Input: part model. Units: mm. Frame: model coordinates. Face numbers are marked on the shaded views. A direction names the side the tool comes from. Round coordinates to 2 decimals unless told otherwise and drop trailing zeros. Write each loop counter-clockwise with the first axis right and the second up, starting at its lowest first coordinate (ties: lowest second). Pieces come first, ordered by that corner, then holes. Notation, with made-up numbers: (75.25, 61) - (102.25, 61) arc R13 cw to (102.25, 69) - close; hole circle Ø5 at (22, 51.25). An arc over 180 degrees is marked (long way). Use one line per item in the form item = value.
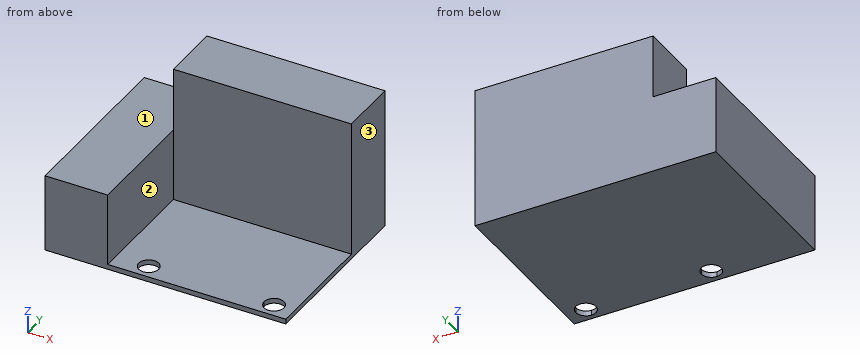
```python
from build123d import *

# Parameters (mm, degrees)
F1_DEPTH = 14.5
F0_W     = 35.5
F0_H     = 12
F2_DEPTH = 27.2
F3_DEPTH = 1


with BuildPart() as f1:
    # F0 (on Top) → F1 (new body)
    with BuildSketch(Plane.XY):
        Polygon((-24, -17.75), (-11.5, -17.75), (-11.5, -16.75), (-11.5, 5.75), (-11.5, 17.75), (-24, 17.75), align=None)
    extrude(amount=F1_DEPTH)

    # F0 (on Top) → F2 (join)
    with BuildSketch(Plane.XY):
        with Locations((6.25, 11.75)):
            Rectangle(F0_W, F0_H)
    extrude(amount=F2_DEPTH)

    # F0 (on Top) → F3 (join)
    with BuildSketch(Plane.XY):
        with Locations((6.25, 11.75)):
            Rectangle(F0_W, F0_H)
        Polygon((-11.5, -17.75), (24, -17.75), (24, -16.75), (20, -16.75), (-5, -16.75), (-11.5, -16.75), align=None)
        Polygon((-24, -17.75), (-11.5, -17.75), (-11.5, -16.75), (-11.5, 5.75), (-11.5, 17.75), (-24, 17.75), align=None)
        with BuildLine():
            Line((-11.5, 5.75), (-11.5, -16.75))
            Line((-11.5, -16.75), (-5, -16.75))
            ThreePointArc((-5, -16.75), (-6.4142135624, -13.3357864376), (-3, -14.75))
            Line((-3, -14.75), (18, -14.75))
            ThreePointArc((18, -14.75), (20, -12.75), (22, -14.75))
            Line((22, -14.75), (24, -14.75))
            Line((24, -14.75), (24, 5.75))
            Line((24, 5.75), (-11.5, 5.75))
        make_face()
        with BuildLine():
            Line((-5, -16.75), (20, -16.75))
            ThreePointArc((20, -16.75), (18.5857864376, -16.1642135624), (18, -14.75))
            Line((18, -14.75), (-3, -14.75))
            ThreePointArc((-3, -14.75), (-3.5857864376, -16.1642135624), (-5, -16.75))
        make_face()
        with BuildLine():
            Line((20, -16.75), (24, -16.75))
            Line((24, -16.75), (24, -14.75))
            Line((24, -14.75), (22, -14.75))
            ThreePointArc((22, -14.75), (21.4142135624, -16.1642135624), (20, -16.75))
        make_face()
    extrude(amount=-F3_DEPTH)


solid = f1.part
```
(1) First-contact query: pin 1 Ø3 at (x, z) = (-7, 22.5) entering from -Y; pin 2 Ø13 at (y, z) = (14.5, 23) entering from -X; pin 3 Ø7 at (y, z) = (-7.5, 9) entering from +X. Flat tips, straight axial feed; report the tip coordinate or a pass-through.
Derived:
pin_1 = 5.75
pin_2 = -11.5
pin_3 = -11.5
(2) Cut plane A-A on y = -10. Output: boundary loops of the cut face in (x, z), then the cut area to 3 significant figures.
Derived:
outline = (-24, -1) - (24, -1) - (24, 0) - (-11.5, 0) - (-11.5, 14.5) - (-24, 14.5) - close
area = 229 mm^2
(3) Cut plane D-D on x = -20. Output: boundary loops of the cut face in (y, z).
Derived:
outline = (-17.75, -1) - (17.75, -1) - (17.75, 14.5) - (-17.75, 14.5) - close
(4) Access query for the marked faces 1, 2 and 3. Directions: +Z, -Z, +X, -X, +Y, -Y. A direction counts if a zero-diameter tool reaches every point of the face in a straight line with its end or side. Return the directions, or none.
Derived:
face_1 = +Z, -X, +Y, -Y
face_2 = +Z, +X, -Y
face_3 = +Z, -Z, +X, +Y, -Y
(5) Cut plane C-C on z = 22.5. Output: boundary loops of the cut face in (x, y).
Derived:
outline = (-11.5, 5.75) - (24, 5.75) - (24, 17.75) - (-11.5, 17.75) - close
(6) Material intervals for L1, parallel to X at y = -14.75, z = -0.45; L2, parallel to Y at x = -5, z = -0.25; L3, parallel to X at y = -2, z = 10.5, sorted ascending.
Derived:
L1 = -24 to -7, -3 to 18, 22 to 24
L2 = -17.75 to -16.75, -12.75 to 17.75
L3 = -24 to -11.5
(7) Cut plane B-B on x = 4. Output: boundary loops of the cut face in (y, z).
Derived:
outline = (-17.75, -1) - (17.75, -1) - (17.75, 27.2) - (5.75, 27.2) - (5.75, 0) - (-17.75, 0) - close
